from build123d import *

# Parameters (mm, degrees)
CROQUIS1_W              = 2.5
CROQUIS1_H              = 13
CORTAR_EXTRUIR1_DEPTH   = 12
CROQUIS4_R              = 2.25
CROQUIS4_R_2            = 0.9
CROQUIS4_W              = 18
CROQUIS4_H              = 1
SALIENTE_EXTRUIR1_DEPTH = 5


with BuildPart() as part:
    # Croquis1 → Revolución1 (revolve)
    with BuildSketch(Plane.XY):
        with Locations((-1.25, 37)):
            Rectangle(CROQUIS1_W, CROQUIS1_H)
        Polygon((-12, -30.5), (0, -30.5), (0, 30.5), (-6.5, 30.5), (-6.5, 26.5), (-9.15, 26.5), (-9.15, 23.5), (-13.65, 23.5), (-13.65, -0.5), (-12, -0.5), align=None)
    revolve(axis=Axis((0, 65.687156563, 0), (0, -1, 0)))

    # Croquis2 → Cortar-Extruir1 (cut)
    with BuildSketch(Plane(origin=(0, 43.5, 0), x_dir=(1, 0, 0), z_dir=(0, 1, 0))):
        Polygon((-55.580517034, 0.96), (-2.308332732, 0.96), (2.308332732, 0.96), (55.580517034, 0.96), (55.580517034, 107.504368605), (-55.580517034, 107.504368605), align=None)
    extrude(amount=-CORTAR_EXTRUIR1_DEPTH, mode=Mode.SUBTRACT)

    # Croquis4 → Saliente-Extruir1 (add)
    with BuildSketch(Plane(origin=(0, 23.5, 0), x_dir=(1, 0, 0), z_dir=(0, 1, 0))):
        with Locations((-10.04, 0)):
            Circle(CROQUIS4_R)
        with Locations((-10.04, 0)):
            Circle(CROQUIS4_R_2, mode=Mode.SUBTRACT)
        with Locations((10.04, 0)):
            Circle(CROQUIS4_R)
        with Locations((10.04, 0)):
            Circle(CROQUIS4_R_2, mode=Mode.SUBTRACT)
        Rectangle(CROQUIS4_W, CROQUIS4_H)
    extrude(amount=SALIENTE_EXTRUIR1_DEPTH)


solid = part.part
Read the model definition and answer for the solid it produces. Units are mm, in the model's axes. A direction names the side the tool comes from. Coordinates: 2 decimals unless noted, no trailing zeros. Loops run counter-clockwise (first coordinate to the right, second up) from the corner with the lowest first, then second, coordinate; pieces in that order, holes last. Notation, with made-up numbers: (9.5, 56.5) -> (66.5, 56.5) arc R25 cw to (66.5, 93.5) -> close; hole circle Ø10 at (30.5, -37). An arc over 180 degrees is marked (long way). Write item = value, one per line. Start each with the question number.
1) The part is cut by section A-A, the plane x = 0. Determine the outline of the cut face in (y, z), plus the area to 3 significant figures.
2) The mould has two halves that part along X. Classify faces 1 (the face through (0.54, 37.09, 2.44)), 2 (the face through (0, -30.5, 0)), 3 (the face through (-10, 23.5, 0)): pulls with the +X half, pulls with the -X half, needs draft (parallel to the pull), parting line crosses it, or undercut.
3) The part is cut by section C-C, the plane y = -5. Determine the outline of the cut face in (x, z), plus the area to 3 significant figures.
4) The part is cut by section D-D, the plane z = -7.5. Determine the outline of the cut face in (x, y).
5) Find the intervals of material crossed by L1, parallel to X at y = 25.65, z = 0; L2, parallel to Z at x = 10.04, y = 27.2; L3, parallel to Y at x = 7.5, z = 7.5, in increasing order. Write a range as from..to.
6) The part is cut by section B-B, the plane z = 4. Determine the outline of the cut face in (x, y).
7) For faces 4 (the face through (0, 38, -0.96)), 5 (the face through (7, 27, 0.5)), 6 (the face through (-9.209, 25.965, 0.345)), 7 (the face through (0, 26.5, -7)), 8 (the face through (-5, -0.5, 11.1)), determine the directions among +Z, -Z, +X, -X, +Y, -Y from which every point of the face is accessible in a straight line to the end or side of a thin tool.
8) Given P1, Ø4, axis at x = 5.5, z = -3, coming from the +Y side; P2, Ø2, axis at x = -5.5, y = -11, coming from the +Z side; P3, Ø0.7, axis at x = 7, y = 27, coming from the -Z side; P4, Ø9.5, axis at x = -4, z = 3.5, coming from the +Y side, each flat-ended and moving along its own axis, determine where each tip first touches the part or whether it passes through.
Result:
q1.outline = (-30.5, -12) -> (-0.5, -12) -> (-0.5, -13.65) -> (23.5, -13.65) -> (23.5, -9.15) -> (26.5, -9.15) -> (26.5, -6.5) -> (30.5, -6.5) -> (30.5, -2.5) -> (31.5, -2.5) -> (31.5, -0.96) -> (43.5, -0.96) -> (43.5, 2.5) -> (30.5, 2.5) -> (30.5, 6.5) -> (26.5, 6.5) -> (26.5, 9.15) -> (23.5, 9.15) -> (23.5, 13.65) -> (-0.5, 13.65) -> (-0.5, 12) -> (-30.5, 12) -> close
q1.area = 1,530 mm²
q2.face_1 = parting line crosses it
q2.face_2 = needs draft
q2.face_3 = undercut
q3.outline = circle Ø24 at (0, 0)
q3.area = 452 mm²
q4.outline = (-11.4, -0.5) -> (-9.37, -0.5) -> (-9.37, -30.5) -> (9.37, -30.5) -> (9.37, -0.5) -> (11.4, -0.5) -> (11.4, 23.5) -> (5.24, 23.5) -> (5.24, 26.5) -> (-5.24, 26.5) -> (-5.24, 23.5) -> (-11.4, 23.5) -> close
q5.L1 = -12.29..-10.94, -9.15..9.15, 10.94..12.29
q5.L2 = -2.25..-0.9, 0.9..2.25
q5.L3 = -30.5..23.5
q6.outline = (-13.05, -0.5) -> (-11.31, -0.5) -> (-11.31, -30.5) -> (11.31, -30.5) -> (11.31, -0.5) -> (13.05, -0.5) -> (13.05, 23.5) -> (8.23, 23.5) -> (8.23, 26.5) -> (5.12, 26.5) -> (5.12, 30.5) -> (-5.12, 30.5) -> (-5.12, 26.5) -> (-8.23, 26.5) -> (-8.23, 23.5) -> (-13.05, 23.5) -> close
q7.face_4 = -Z, +X, -X, +Y
q7.face_5 = +Z, +Y
q7.face_6 = +Y
q7.face_7 = -Z, +Y
q7.face_8 = -Y
q8.P1 = 30.5
q8.P2 = 11.12
q8.P3 = -0.5
q8.P4 = 43.5
